Verification items for the finished model (mm, model axes). Face numbers are marked on the shaded views. A direction names the side the tool comes from. Round coordinates to 2 decimals unless told otherwise and drop trailing zeros. Write each loop counter-clockwise with the first axis right and the second up, starting at its lowest first coordinate (ties: lowest second). Pieces come first, ordered by that corner, then holes. Notation, with made-up numbers: (-25, 5) - (32, 5) arc R17 ccw to (32, 26) - close; hole circle Ø7 at (-12, 88). An arc over 180 degrees is marked (long way). Answer as a JSON object with one key per item and string values. Group by question number.
1) Set-up check for the marked faces 1, 2 and 3: record each of +Z, -Z, +X, -X, +Y, -Y from which the full face is reachable in a straight line by a thin tool's end or side.
2) Section check C-C (z = 15.5). Enter the section's corners in (x, y), then the cut area to 3 significant figures.
3) Section check B-B (y = -3). Enter the section's corners in (x, z).
4) Go/stop test with flat-tipped pins: pin 1 Ø10 at (y, z) = (8.5, 87.5) entering from +X; pin 2 Ø2 at (x, z) = (7, 107.5) entering from +Y; pin 3 Ø1 at (y, z) = (15.5, 62.5) entering from +X. Record where each tip stops, or that it passes through.
5) Thickness scan on line 1 (Z direction, x = -2.5, y = 14.5); line 2 (Y direction, x = -0.5, z = 43). Record the ranges inside material, lowest first.
6) Section check D-D (z = 86). Enter the section's corners in (x, y), then the cut area to 3 significant figures.
7) Section check A-A (x = 0). Enter the section's corners in (y, z).
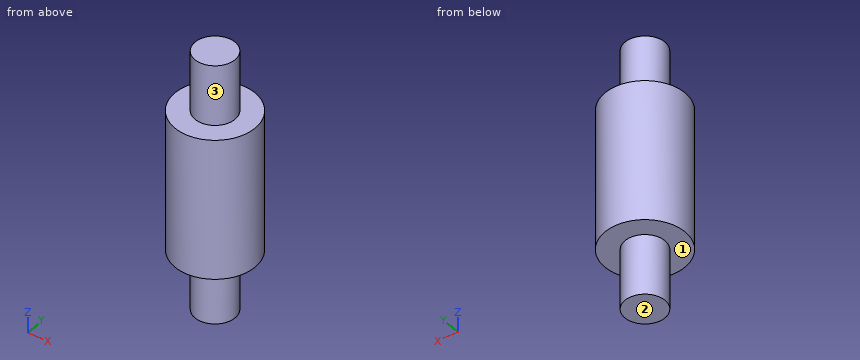
```python
from build123d import *

# Parameters (mm, degrees)
SKETCH2_R           = 20
BOSS_EXTRUDE4_DEPTH = 130
SKETCH3_OUTSIDE_W   = 70.354
SKETCH3_OUTSIDE_H   = 70.354
SKETCH3_OUTSIDE_R   = 10
CUT_EXTRUDE1_DEPTH  = 30
SKETCH4_OUTSIDE_W   = 70.354
SKETCH4_OUTSIDE_H   = 70.354
SKETCH4_OUTSIDE_R   = 10
CUT_EXTRUDE2_DEPTH  = 30


with BuildPart() as part:
    # Sketch2 → Boss-Extrude4 (new body)
    with BuildSketch(Plane.XY):
        Circle(SKETCH2_R)
    extrude(amount=BOSS_EXTRUDE4_DEPTH)

    # Sketch3 outside → Cut-Extrude1 (cut)
    with BuildSketch(Plane.XY.offset(130)):
        Rectangle(SKETCH3_OUTSIDE_W, SKETCH3_OUTSIDE_H)
        Circle(SKETCH3_OUTSIDE_R, mode=Mode.SUBTRACT)
    extrude(amount=-CUT_EXTRUDE1_DEPTH, mode=Mode.SUBTRACT)

    # Sketch4 outside → Cut-Extrude2 (cut)
    with BuildSketch(Plane(origin=(0, 0, 0), x_dir=(-1, 0, 0), z_dir=(0, 0, -1))):
        Rectangle(SKETCH4_OUTSIDE_W, SKETCH4_OUTSIDE_H)
        Circle(SKETCH4_OUTSIDE_R, mode=Mode.SUBTRACT)
    extrude(amount=-CUT_EXTRUDE2_DEPTH, mode=Mode.SUBTRACT)


solid = part.part
```
Returned:
{
 "1": {"face 1": "-Z", "face 2": "-Z, +X, -X, +Y, -Y", "face 3": "+Z"},
 "2": {"outline": "circle Ø20 at (0, 0)", "area": "314 mm2"},
 "3": {"outline": "(-19.77, 30) - (-9.54, 30) - (-9.54, 0) - (9.54, 0) - (9.54, 30) - (19.77, 30) - (19.77, 100) - (9.54, 100) - (9.54, 130) - (-9.54, 130) - (-9.54, 100) - (-19.77, 100) - close"},
 "4": {"pin 1": "x = 19.69", "pin 2": "y = 8", "pin 3": "x = 13.23"},
 "5": {"line 1": "30 to 100", "line 2": "-19.99 to 19.99"},
 "6": {"outline": "circle Ø40 at (0, 0)", "area": "1,260 mm2"},
 "7": {"outline": "(-20, 30) - (-10, 30) - (-10, 0) - (10, 0) - (10, 30) - (20, 30) - (20, 100) - (10, 100) - (10, 130) - (-10, 130) - (-10, 100) - (-20, 100) - close"}
}
